Autodesk Inventor part; units mm, degrees
ref_plane "YZ Plane" through (0, 0, 0) normal (1, 0, 0) x (0, 1, 0)
ref_plane "XZ Plane" through (0, 0, 0) normal (0, 1, 0) x (-1, 0, 0)
ref_plane "XY Plane" through (0, 0, 0) normal (0, 0, 1) x (1, 0, 0)
sketch "Boceto1" plane through (0, 0, 0) normal (0, 0, 1) x (1, 0, 0)
  circle A0 centre (0, 0) radius 1.5
  arc A1 (0, 2.3) -> (1.15, 1.9919) centre (0, 0) ccw
  line L0 (-2.3, 0) -> (-2.3, 11)
  line L1 (0, -2.3) -> (0, 17.0308) construction
  circle A2 centre (-0.3, 11) radius 2
  line L2 (0.9, 7) -> (0.9, 2.4249)
  line L3 (-6.6108, 0) -> (6.6108, 0) construction
  arc A3 (3.9, 10) -> (0.9, 7) centre (3.9, 7) ccw
  line L4 (-2.4885, 11) -> (5.8935, 11) construction
  line L5 (0.8529, 10) -> (0.9, 10)
  line L6 (3.9, 10) -> (5.7216, 10)
  line L7 (0.656, 12.7567) -> (5.7248, 9.9983)
  arc A4 (0.9, 2.4249) -> (1.15, 1.9919) centre (1.4, 2.4249) ccw
  point P0 (0.9, 2.1166)
  dimension "d3" = 4
  dimension "d0" = 2.3
  dimension "d1" = 3
  dimension "d2" = 11
  dimension "d5" = 3.2
  dimension "d6" = 6
  dimension "d7" = 11
  dimension "d9" = 10
  dimension "d21" = 1
extrude "Extrusión1" add sketch "Boceto1" along normal mid plane 2
sketch "Boceto2" plane through (-2.3, 0, 1) normal (-1, 0, 0) x (0, 0, 1)
  line L0 (-1, 0) -> (-1, 11) construction
  line L1 (-2, 11) -> (0, 11)
  line L2 (-2, 0) -> (0, 0)
  line L3 (0, 11) -> (0, 0)
  line L4 (-2, 11) -> (0, 11)
  line L5 (-2, 0) -> (-2, 11)
  circle A0 centre (-1, 9) radius 0.5
  dimension "d12" = 1
  dimension "d13" = 9
hole "Agujero1" at (-2.3, 9, 0) direction (1, 0, 0) diameter 1 depth 2.3
properties part number "Hudson 1-62D"
CAD build for the part. Positions are in the model's coordinates, mm. A direction names the side the tool comes from. Coordinates: 2 decimals unless noted, no trailing zeros. Order: outer loops, then holes, each group sorted by start corner. A loop starts at its lowest first (then second) coordinate and runs counter-clockwise, first axis right, second up. Notation, with made-up numbers: M -39,-9.5 L -22,-9.5 A6 cw -22,-1.5 Z; hole C 69.5,82 d7. An arc over 180 degrees is marked long. Write each question's results on one line, items separated by ' | '. Start each with the question number.
Q1. Drill centre lines: probe 1 along Z at (x, y) = (-1.4, 9); probe 2 along Y at (x, z) = (-1.35, 0); probe 3 along X at (y, z) = (6.5, -0.5). Where is each one in solid material? Low to high. Write a range as from..to.
Q2. Flat gauge pins, fed straight in: P1, Ø1, axis at x = 1, y = 7, coming from the +Z side; P2, Ø0.5, axis at y = 9, z = 0, coming from the -X side. Where does each tip first touch, or does it go through?
Q3. Cut at A-A (z = -0.3). List the corners of the cut face in (x, y), then the cut area to 3 significant figures.
Q4. Cut at C-C (y = 9). List the corners of the cut face in (x, z).
Q5. Pull direction Z, two halves, no side cores. Call faces 4 (the cylindrical face through (-1.35, 12.7, -0.01)), 5 (the flat face through (0, 9, 0)), 6 (the flat face through (0, 7, -1)): +Z half, -Z half, draft (parallel to the pull), parting line (faces both ways), or undercut.
Q6. Cut at D-D (y = 5.25). List the corners of the cut face in (x, z), then the cut area to 3 significant figures.
Q7. Which spindle directions (+Z, -Z, +X, -X, +Y, -Y) get a long thin tool onto all of the face, cutting with end or side? Do faces 1 (the flat face through (5, 10, 0)), 2 (the flat face through (0.9, 5, 0)), 3 (the cylindrical face through (-1.134, 9.488, -0.108)). Say none if no direction does.
Q8. Cut at B-B (x = 0.25). List the corners of the cut face in (y, z), then the cut area to 3 significant figures.
Found:
1) probe 1: -1..-0.5, 0.5..1 | probe 2: -1.86..-0.65, 0.65..8.5, 9.5..12.7 | probe 3: -2.3..0.9
2) P1: z = 1 | P2: x = 0
3) outline: M -2.3,0 A2.3 ccw long 1.15,1.99 A0.5 cw 0.9,2.42 L 0.9,7 A3 cw 3.9,10 L 5.72,10 L 0.66,12.76 A2 ccw -2.3,11 L -2.3,9.4 L 0,9.4 L 0,8.6 L -2.3,8.6 Z; hole C 0,0 d3 | area: 50.4 mm²
4) outline: M -2.3,-1 L 1.66,-1 L 1.66,1 L -2.3,1 L -2.3,0.5 L 0,0.5 L 0,-0.5 L -2.3,-0.5 Z
5) face 4: draft | face 5: undercut | face 6: -Z half
6) outline: M -2.3,-1 L 0.9,-1 L 0.9,1 L -2.3,1 Z | area: 6.40 mm²
7) face 1: +Z, -Z, +X, -Y | face 2: +Z, -Z, +X | face 3: -X
8) outline: M -2.29,-1 L -1.48,-1 L -1.48,1 L -2.29,1 Z; M 1.48,-1 L 12.92,-1 L 12.92,1 L 1.48,1 Z | area: 24.5 mm²
